from build123d import *

# Parameters (mm, degrees)
SKETCH1_R           = 12.7
BOSS_EXTRUDE1_DEPTH = 177.8
SKETCH4_R           = 10.414
BOSS_EXTRUDE2_DEPTH = 5.08
SKETCH5_R           = 7.874
CUT_EXTRUDE1_DEPTH  = 184.759828036
SKETCH6_R           = 10.287
SKETCH6_R_2         = 7.874
BOSS_EXTRUDE3_DEPTH = 12.7


with BuildPart() as part:
    # Sketch1 → Boss-Extrude1 (new body)
    with BuildSketch(Plane(origin=(0, 0, 0), x_dir=(1, 0, 0), z_dir=(0, 1, 0))):
        with Locations(Location((0, 0, 0), (0, 0, 270))):
            Circle(SKETCH1_R)
    extrude(amount=BOSS_EXTRUDE1_DEPTH)

    # Sketch4 → Boss-Extrude2 (add)
    with BuildSketch(Plane(origin=(0, 177.8, 0), x_dir=(1, 0, 0), z_dir=(0, 1, 0))):
        with Locations(Location((0, 0, 0), (0, 0, 270))):
            Circle(SKETCH4_R)
    extrude(amount=BOSS_EXTRUDE2_DEPTH)

    # Sketch5 → Cut-Extrude1 (cut, through all)
    with BuildSketch(Plane(origin=(0, 182.88, 0), x_dir=(1, 0, 0), z_dir=(0, 1, 0))):
        with Locations(Location((0, 0, 0), (0, 0, 270))):
            Circle(SKETCH5_R)
    extrude(amount=-CUT_EXTRUDE1_DEPTH, mode=Mode.SUBTRACT)

    # Sketch6 → Boss-Extrude3 (add)
    with BuildSketch(Plane.XZ):
        with Locations(Location((0, 0, 0), (0, 0, 90))):
            Circle(SKETCH6_R)
        with Locations(Location((0, 0, 0), (0, 0, 90))):
            Circle(SKETCH6_R_2, mode=Mode.SUBTRACT)
    extrude(amount=BOSS_EXTRUDE3_DEPTH)


solid = part.part
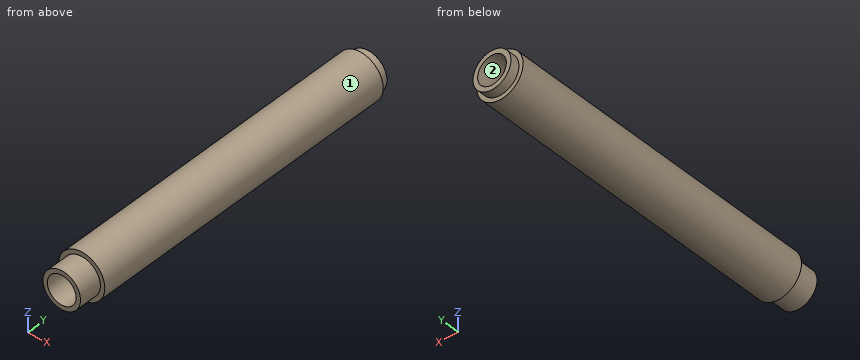
Could you check a few things on this model? Use its own coordinates, in mm. Face numbers are marked on the shaded views. Round coordinates to 2 decimals unless told otherwise and drop trailing zeros. Write each loop counter-clockwise with the first axis right and the second up, starting at its lowest first coordinate (ties: lowest second). Pieces come first, ordered by that corner, then holes. Notation, with made-up numbers: (-15, 1.5) - (19, 1.5) arc R15 ccw to (19, 16.5) - close; hole circle Ø8 at (-24, 87.5). An arc over 180 degrees is marked (long way). Put each result on its own line as item: value. Start each with the question number.
(1) Thinking about a two-plate mould opening in X: for the marked faces 1 and 2, which applies, released by +X, released by -X, zero draft, split by the parting line, or undercut?
(2) I want a section at B-B, the plane z = 0. Please give me the cut outline in (x, y).
(3) I want a section at A-A, the plane x = 0. Please give me the cut outline in (y, z).
(4) Will these pins go through, and if not, where does the flat tip stop? pin 1 (1 mm diameter, centred on x = 6, y = 29, fed in from -Z); pin 2 (8 mm diameter, centred on x = -8, y = 37.5, fed in from +Z); pin 3 (4 mm diameter, centred on y = 77.5, z = 7.5, fed in from +X).
(5) I want a section at C-C, the plane y = 68.5. Please give me the cut outline in (x, z).
(6) I need wall thicknesses on probe 1 along X at (y, z) = (93, 0); probe 2 along X at (y, z) = (12, 0.75); probe 3 along Z at (x, y) = (4.75, 29). Which ranges of each line are inside material? Lowest first, please.
Here are the results:
1. face 1: split by the parting line
1. face 2: undercut
2. outline: (-12.7, 0) - (-10.29, 0) - (-10.29, -12.7) - (-7.87, -12.7) - (-7.87, 182.88) - (-10.41, 182.88) - (-10.41, 177.8) - (-12.7, 177.8) - close; (7.87, -12.7) - (10.29, -12.7) - (10.29, 0) - (12.7, 0) - (12.7, 177.8) - (10.41, 177.8) - (10.41, 182.88) - (7.87, 182.88) - close
3. outline: (-12.7, -10.29) - (0, -10.29) - (0, -12.7) - (177.8, -12.7) - (177.8, -10.41) - (182.88, -10.41) - (182.88, -7.87) - (-12.7, -7.87) - close; (-12.7, 7.87) - (182.88, 7.87) - (182.88, 10.41) - (177.8, 10.41) - (177.8, 12.7) - (0, 12.7) - (0, 10.29) - (-12.7, 10.29) - close
4. pin 1: stops at z = -11.45
4. pin 2: stops at z = 12.05
4. pin 3: stops at x = 11.45
5. outline: circle Ø25.4 at (0, 0); hole circle Ø15.75 at (0, 0)
6. probe 1: x = -12.7 to -7.87, 7.87 to 12.7
6. probe 2: x = -12.68 to -7.84, 7.84 to 12.68
6. probe 3: z = -11.78 to -6.28, 6.28 to 11.78
